Check sheet for the modelled part. Datum: model origin and axes. Units: mm. Face numbers are marked on the shaded views. A direction names the side the tool comes from. Give positions to 0.01 mm unless a question says otherwise; leave off trailing zeros. Loops run counter-clockwise (first coordinate to the right, second up) from the corner with the lowest first, then second, coordinate; pieces in that order, holes last. Notation, with made-up numbers: (84, 63.25) - (110, 63.25) arc R26 ccw to (110, 84.25) - close; hole circle Ø1 at (4, 82.25). An arc over 180 degrees is marked (long way). Answer in a Markdown table with one row per item. Add a question column.
(1) Thickness scan on L1, parallel to X at y = 5, z = 0; L2, parallel to Z at x = -4, y = 1.25; L3, parallel to Z at x = -11, y = 7.75. Record the ranges inside material, lowest first.
(2) Go/stop test with flat-tipped pins: P1, Ø1.2, axis at y = 4.5, z = 10.5, coming from the +X side; P2, Ø0.8, axis at y = 6, z = 11, coming from the -X side; P3, Ø8, axis at x = -12, z = -12.5, coming from the -Y side; P4, Ø1, axis at x = 10, z = -2.5, coming from the +Y side. Record where each tip stops, or that it passes through.
(3) Sectioned sample at A-A on y = 7. State how many separate pieces and enclosed holes the cut face has, then the cut area to 3 significant figures.
(4) Set-up check for the marked faces 5, 6 and 7: record each of +Z, -Z, +X, -X, +Y, -Y from which the full face is reachable in a straight line by a thin tool's end or side.
(5) Sectioned sample at C-C on y = -3.5. Enter the section's corners in (x, z), then the cut area to 3 significant figures.
(6) Draft check along Z on the marked faces 1, 2, 3 and 4. Enter one of: released by +Z, released by -Z, zero draft, split by the parting line, or undercut.
from build123d import *
from OCP.BRepFilletAPI import BRepFilletAPI_MakeChamfer

# Parameters (mm, degrees)
SKETCH_1_R          = 17
SKETCH_1_R_2        = 1.4
EXTRUDE_1_DEPTH     = 8
SKETCH_2_W          = 2
SKETCH_2_H          = 5
SKETCH_5_R          = 1.4
CUT_EXTRUDE_3_DEPTH = 6
SKETCH_6_R          = 8.5
EXTRUDE_2_DEPTH     = 6
SKETCH_4_R          = 3
CUT_EXTRUDE_2_DEPTH = 28.820855486
SKETCH_7_R          = 9.5
SKETCH_7_R_2        = 8.5
EXTRUDE_3_DEPTH     = 1
CHAMFER_1_SIZE      = 2.383507185
CHAMFER_1_SIZE_2    = 2
FILLET_1_R          = 0.5
CUT_EXTRUDE_START   = -10
CUT_EXTRUDE_4_DEPTH = 10
FILLET_2_R          = 1
CHAMFER_2_SIZE      = 0.5
CHAMFER_2_SIZE2     = 0.595876796


with BuildPart() as part:
    # 草图1 → 凸台-拉伸1 (new body)
    # profile 1 of 5: a face of its own
    with BuildSketch(Plane(origin=(0, 0, 0), x_dir=(1, 0, 0), z_dir=(0, 1, 0))):
        with Locations(Location((0, 0, 0), (0, 0, 270))):
            Circle(SKETCH_1_R)
        with Locations((-7, 0)):
            Circle(SKETCH_1_R_2, mode=Mode.SUBTRACT)
        with Locations((0, -7)):
            Circle(SKETCH_1_R_2, mode=Mode.SUBTRACT)
        with Locations((7, 0)):
            Circle(SKETCH_1_R_2, mode=Mode.SUBTRACT)
        with Locations((0, 7)):
            Circle(SKETCH_1_R_2, mode=Mode.SUBTRACT)
    # profile 2 of 5: a face of its own
    with BuildSketch(Plane(origin=(0, 0, 0), x_dir=(1, 0, 0), z_dir=(0, 1, 0))):
        with Locations((0, 7)):
            Circle(SKETCH_1_R_2)
    # profile 3 of 5: a face of its own
    with BuildSketch(Plane(origin=(0, 0, 0), x_dir=(1, 0, 0), z_dir=(0, 1, 0))):
        with Locations((-7, 0)):
            Circle(SKETCH_1_R_2)
    # profile 4 of 5: a face of its own
    with BuildSketch(Plane(origin=(0, 0, 0), x_dir=(1, 0, 0), z_dir=(0, 1, 0))):
        with Locations((0, -7)):
            Circle(SKETCH_1_R_2)
    # profile 5 of 5: a face of its own
    with BuildSketch(Plane(origin=(0, 0, 0), x_dir=(1, 0, 0), z_dir=(0, 1, 0))):
        with Locations((7, 0)):
            Circle(SKETCH_1_R_2)
    extrude(amount=EXTRUDE_1_DEPTH)

    # 草图2 → 切除-旋转1 (revolve, cut)
    with BuildSketch(Plane.XY, mode=Mode.PRIVATE) as cut_revolve_1_sk:
        with Locations((16, 4)):
            Rectangle(SKETCH_2_W, SKETCH_2_H)
    revolve(cut_revolve_1_sk.sketch.rotate(Axis((0, 8, 0), (0, -1, 0)), 90), axis=Axis((0, 8, 0), (0, -1, 0)), mode=Mode.SUBTRACT)

    # 草图5 → 切除-拉伸3 (cut)
    with BuildSketch(Plane(origin=(0, 8, 0), x_dir=(1, 0, 0), z_dir=(0, 1, 0))):
        with Locations(Location((0, 7, 0), (0, 0, 270))):
            Circle(SKETCH_5_R)
        with Locations(Location((7, 0, 0), (0, 0, 270))):
            Circle(SKETCH_5_R)
        with Locations(Location((0, -7, 0), (0, 0, 270))):
            Circle(SKETCH_5_R)
        with Locations(Location((-7, 0, 0), (0, 0, 270))):
            Circle(SKETCH_5_R)
    extrude(amount=-CUT_EXTRUDE_3_DEPTH, mode=Mode.SUBTRACT)

    # 草图6 → 凸台-拉伸2 (add)
    with BuildSketch(Plane.XZ):
        with Locations(Location((0, 0, 0), (0, 0, 270))):
            Circle(SKETCH_6_R)
    extrude(amount=EXTRUDE_2_DEPTH)

    # 草图4 → 切除-拉伸2 (cut, through all)
    with BuildSketch(Plane(origin=(0, 8, 0), x_dir=(1, 0, 0), z_dir=(0, 1, 0))):
        with Locations(Location((0, 0, 0), (0, 0, 270))):
            Circle(SKETCH_4_R)
    extrude(amount=-CUT_EXTRUDE_2_DEPTH, mode=Mode.SUBTRACT)

    # 草图7 → 凸台-拉伸3 (add)
    with BuildSketch(Plane.XZ):
        with Locations(Location((0, 0, 0), (0, 0, 90))):
            Circle(SKETCH_7_R)
        with Locations(Location((0, 0, 0), (0, 0, 270))):
            Circle(SKETCH_7_R_2, mode=Mode.SUBTRACT)
    extrude(amount=EXTRUDE_3_DEPTH)

    # 倒角1
    chamfer_1_edges_1 = [part.edges().sort_by_distance(p)[0] for p in [
        (0, 6.5, -15),
    ]]
    chamfer_1_side_1 = [part.faces().sort_by_distance(p)[0] for p in [
        (0, 6.46, -15),
    ]]
    chamfer_1_edges_2 = [part.edges().sort_by_distance(p)[0] for p in [
        (0, 1.5, -15),
    ]]
    chamfer_1_side_2 = [part.faces().sort_by_distance(p)[0] for p in [
        (0, 1.5, -15.04),
    ]]
    chamfer_1 = BRepFilletAPI_MakeChamfer(part.part.solid().wrapped)
    for e in chamfer_1_edges_1:
        chamfer_1.Add(CHAMFER_1_SIZE - 0.0001, CHAMFER_1_SIZE_2 - 0.0001, e.wrapped, chamfer_1_side_1[0].wrapped)
    for e in chamfer_1_edges_2:
        chamfer_1.Add(CHAMFER_1_SIZE_2 - 0.0001, CHAMFER_1_SIZE - 0.0001, e.wrapped, chamfer_1_side_2[0].wrapped)
    add(Compound.cast(chamfer_1.Shape()), mode=Mode.REPLACE)  # a hair under: the kernel refuses the full size

    # 圆角1
    fillet_1_edges = [part.edges().sort_by_distance(p)[0] for p in [
        (0, -6, 8.5),
    ]]
    fillet(fillet_1_edges, radius=FILLET_1_R)

    # 草图8 → 切除-拉伸4 (cut)
    with BuildSketch(Plane.XZ.offset(CUT_EXTRUDE_START)):
        with BuildLine():
            Line((-1.5, 9.38083152), (-1.5, 12.91317157))
            ThreePointArc((-1.5, 12.91317157), (-9.192388155, 9.192388155), (-12.91317157, 1.5))
            Line((-12.91317157, 1.5), (-9.38083152, 1.5))
            ThreePointArc((-9.38083152, 1.5), (-6.717514421, 6.717514421), (-1.5, 9.38083152))
        make_face()
        with BuildLine():
            Line((-9.38083152, -1.5), (-12.91317157, -1.5))
            ThreePointArc((-12.91317157, -1.5), (-9.192388155, -9.192388155), (-1.5, -12.91317157))
            Line((-1.5, -12.91317157), (-1.5, -9.38083152))
            ThreePointArc((-1.5, -9.38083152), (-6.717514421, -6.717514421), (-9.38083152, -1.5))
        make_face()
        with BuildLine():
            ThreePointArc((1.5, -12.91317157), (9.192388155, -9.192388155), (12.91317157, -1.5))
            Line((12.91317157, -1.5), (9.38083152, -1.5))
            ThreePointArc((9.38083152, -1.5), (6.717514421, -6.717514421), (1.5, -9.38083152))
            Line((1.5, -9.38083152), (1.5, -12.91317157))
        make_face()
        with BuildLine():
            ThreePointArc((12.91317157, 1.5), (9.192388155, 9.192388155), (1.5, 12.91317157))
            Line((1.5, 12.91317157), (1.5, 9.38083152))
            ThreePointArc((1.5, 9.38083152), (6.717514421, 6.717514421), (9.38083152, 1.5))
            Line((9.38083152, 1.5), (12.91317157, 1.5))
        make_face()
    extrude(amount=CUT_EXTRUDE_4_DEPTH, mode=Mode.SUBTRACT)

    # 圆角2
    fillet_2_edges = [part.edges().sort_by_distance(p)[0] for p in [
        (-1.5, 4, 12.91317157),
        (-1.5, 4, 9.38083152),
        (-9.38083152, 4, 1.5),
        (-12.91317157, 4, 1.5),
        (12.91317157, 4, 1.5),
        (9.38083152, 4, 1.5),
        (1.5, 4, 9.38083152),
        (1.5, 4, 12.91317157),
        (1.5, 4, -12.91317157),
        (1.5, 4, -9.38083152),
        (9.38083152, 4, -1.5),
        (12.91317157, 4, -1.5),
        (-12.91317157, 4, -1.5),
        (-9.38083152, 4, -1.5),
        (-1.5, 4, -9.38083152),
        (-1.5, 4, -12.91317157),
    ]]
    fillet(fillet_2_edges, radius=FILLET_2_R)

    # 倒角2
    chamfer_2_edges = [part.edges().sort_by_distance(p)[0] for p in [
        (0, 8, -8.4),
        (7, 8, -1.4),
        (0, 8, 5.6),
        (-7, 8, -1.4),
    ]]
    chamfer_2_side = [part.faces().sort_by_distance(p)[0] for p in [
        (-10.967366811, 8, 1.019167389),
    ]]
    chamfer(chamfer_2_edges, length=CHAMFER_2_SIZE, length2=CHAMFER_2_SIZE2, reference=chamfer_2_side[0])


solid = part.part
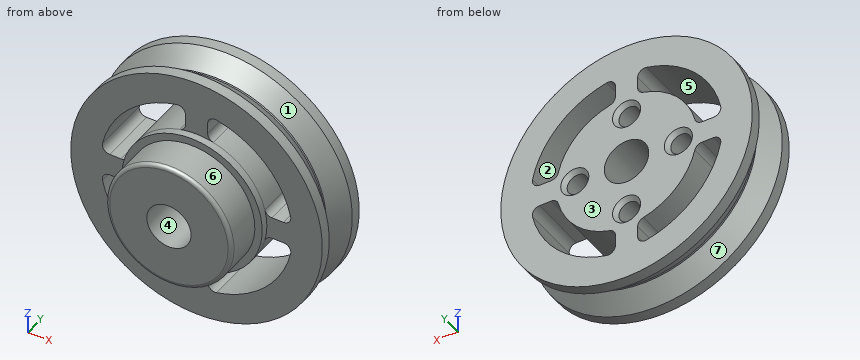
Reply:
| question | item | result |
|---|---|---|
| 1 | L1 | -15.74 to -8.4, -5.6 to -3, 3 to 5.6, 8.4 to 15.74 |
| 1 | L2 | -16.52 to -12.37, -8.62 to 8.62, 12.37 to 16.52 |
| 1 | L3 | -12.96 to -6.93, -1.5 to 1.5, 6.93 to 12.96 |
| 2 | P1 | x = 12.02 |
| 2 | P2 | x = -12.97 |
| 2 | P3 | y = 0 |
| 2 | P4 | through |
| 3 | separate pieces | 1 |
| 3 | enclosed holes | 9 |
| 3 | area | 653 mm^2 |
| 4 | face 5 | +Y, -Y |
| 4 | face 6 | -Y |
| 4 | face 7 | none |
| 5 | outline | circle Ø17 at (0, 0); hole circle Ø6 at (0, 0) |
| 5 | area | 199 mm^2 |
| 6 | face 1 | split by the parting line |
| 6 | face 2 | undercut |
| 6 | face 3 | zero draft |
| 6 | face 4 | undercut |
